from build123d import *

# Parameters (mm, degrees)
SKETCH1_R           = 1.45
BOSS_EXTRUDE1_DEPTH = 8.5
BOSS_EXTRUDE2_START = -8.5
BOSS_EXTRUDE2_DEPTH = 8.5


with BuildPart() as part:
    # Sketch1 → Boss-Extrude1 (new body)
    with BuildSketch(Plane(origin=(0, 0, 0), x_dir=(0, 0, -1), z_dir=(1, 0, 0))):
        with BuildLine():
            Line((27, 10), (5, 10))
            ThreePointArc((5, 10), (0, 5), (5, 0))
            Line((5, 0), (27, 0))
            ThreePointArc((27, 0), (32, 5), (27, 10))
        make_face()
        with Locations((5, 5)):
            Circle(SKETCH1_R, mode=Mode.SUBTRACT)
        with Locations((27, 5)):
            Circle(SKETCH1_R, mode=Mode.SUBTRACT)
    extrude(amount=BOSS_EXTRUDE1_DEPTH)

    # Sketch2 → Boss-Extrude2 (add)
    with BuildSketch(Plane(origin=(8.5, 0, 0), x_dir=(0, 0, -1), z_dir=(1, 0, 0)).offset(BOSS_EXTRUDE2_START)):
        with BuildLine():
            add(Edge.make_bspline(
                [(63.752972286, 17.872423117), (45.928882678, 26.563787963), (31.059268621, 10), (13.694974759, 10)],
                knots=[0, 0, 0, 0, 1, 1, 1, 1], degree=3))
            Line((13.694974759, 10), (27, 10))
            ThreePointArc((27, 10), (31.87285141, 6.120410255), (29.183837075, 0.502127655))
            Line((29.183837075, 0.502127655), (38.08542066, 4.824084077))
            add(Edge.make_bspline(
                [(38.08542066, 4.824084077), (46.797509509, 11.895222457), (57.948000409, 11.067843667)],
                knots=[0, 0, 0, 1, 1, 1], degree=2))
            Line((57.948000409, 11.067843667), (65.313809691, 14.189518476))
            Line((65.313809691, 14.189518476), (63.752972286, 17.872423117))
        make_face()
    extrude(amount=BOSS_EXTRUDE2_DEPTH)


solid = part.part
Could you check a few things on this model? Use its own coordinates, in mm. A direction names the side the tool comes from. Give positions to 0.01 mm unless a question says otherwise; leave off trailing zeros. Order: outer loops, then holes, each group sorted by start corner. A loop starts at its lowest first (then second) coordinate and runs counter-clockwise, first axis right, second up.
1. Will these pins go through, and if not, where does the flat tip stop? P1, Ø5, axis at x = 6.5, z = -32.5, coming from the -Y side; P2, Ø5, axis at x = 5, z = -18, coming from the +Y side; P3, Ø1.5, axis at x = 3, y = 15.5, coming from the +Z side; P4, Ø2.5, axis at y = 5, z = -27, coming from the +X side.
2. We'd pull the mould along Z, two halves only. Please class faces 1 (the cylindrical face through (4.19, 5.06, -3.55)), 2 (the flat face through (0, 11, -32)), 3 (the flat face through (4.19, 16.005, -64.544)): pulls with the +Z half, pulls with the -Z half, needs draft (parallel to the pull), parting line crosses it, or undercut.
3. I need wall thicknesses on L1, parallel to Y at x = 6.5, z = -5; L2, parallel to Y at x = 0.5, z = -9; L3, parallel to Z at x = 6.25, y = 3.75. Which ranges of each line are inside material? Lowest first, please.
4. Suppose I cut it at A-A (x = 3.5). Give the number of separate pieces and of enclosed holes in the cut face, plus the area to 3 significant figures.
5. For faces 4 (the flat face through (4.19, 2.63, -33.57)), 5 (the flat face through (4, 10, -9)), which set-ups out of +Z, -Z, +X, -X, +Y, -Y let a thin tool reach every point of the face, with its end or its side?
6. Suppose I cut it at B-B (z = -8.5). List the corners of the cut face in (x, y) for me, plus the area to 3 significant figures.
Solved:
1. P1: stops at y = 0.9
1. P2: stops at y = 10.78
1. P3: stops at z = -32.38
1. P4: passes through
2. face 1: undercut
2. face 2: needs draft
2. face 3: pulls with the -Z half
3. L1: y = 0 to 3.55, 6.45 to 10
3. L2: y = 0 to 10
3. L3: z = -35.87 to -27.73, -26.27 to -5.73, -4.27 to -0.16
4. separate pieces: 1
4. enclosed holes: 2
4. area: 641 mm2
5. face 4: -Z, +X, -X, -Y
5. face 5: +Z, +X, -X, +Y
6. outline: (0, 0) - (8.5, 0) - (8.5, 10) - (0, 10) - close
6. area: 85.0 mm2
